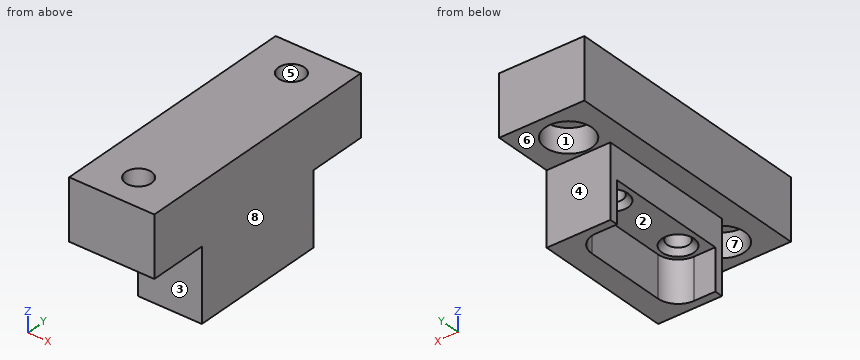
```python
from build123d import *

# Parameters (mm, degrees)
SKETCH2_W           = 16.5
SKETCH2_H           = 50
SKETCH2_R           = 2.5
BOSS_EXTRUDE1_DEPTH = 11.655
CUT_EXTRUDE3_START  = -7
SKETCH4_R           = 4.5
CUT_EXTRUDE3_DEPTH  = 10
SKETCH6_W           = 12.35
SKETCH6_H           = 27
BOSS_EXTRUDE2_DEPTH = 6
SKETCH7_R           = 2.1
CUT_EXTRUDE4_DEPTH  = 6
CHAMFER1_SIZE       = 1
BOSS_EXTRUDE3_DEPTH = 8


with BuildPart() as part:
    # Sketch2 → Boss-Extrude1 (new body)
    with BuildSketch(Plane.XY):
        with Locations((-2.723788813, 9.906715388)):
            Rectangle(SKETCH2_W, SKETCH2_H)
        with Locations((-2.723788813, -8.593284612)):
            Circle(SKETCH2_R, mode=Mode.SUBTRACT)
        with Locations((-2.723788813, 28.406715388)):
            Circle(SKETCH2_R, mode=Mode.SUBTRACT)
    extrude(amount=BOSS_EXTRUDE1_DEPTH)

    # Sketch4 → Cut-Extrude3 (cut)
    with BuildSketch(Plane.XY.offset(11.655).offset(CUT_EXTRUDE3_START)):
        with Locations((-2.723788813, 28.406715388)):
            Circle(SKETCH4_R)
        with Locations((-2.723788813, -8.593284612)):
            Circle(SKETCH4_R)
    extrude(amount=-CUT_EXTRUDE3_DEPTH, mode=Mode.SUBTRACT)

    # Sketch6 → Boss-Extrude2 (add)
    with BuildSketch(Plane(origin=(0, 0, 0), x_dir=(-1, 0, 0), z_dir=(0, 0, -1))):
        with Locations((0.648788813, 9.906715388)):
            Rectangle(SKETCH6_W, SKETCH6_H)
    extrude(amount=BOSS_EXTRUDE2_DEPTH)

    # Sketch7 → Cut-Extrude4 (cut)
    with BuildSketch(Plane(origin=(0, 0, -6), x_dir=(-1, 0, 0), z_dir=(0, 0, -1))):
        with Locations((2.723788813, 17.906715388)):
            Circle(SKETCH7_R)
        with Locations((2.723788813, 1.906715388)):
            Circle(SKETCH7_R)
    extrude(amount=-CUT_EXTRUDE4_DEPTH, mode=Mode.SUBTRACT)

    # Chamfer1
    chamfer1_edges = [part.edges().sort_by_distance(p)[0] for p in [
        (-0.623788813, 17.906715388, -6),
        (-0.623788813, 1.906715388, -6),
    ]]
    chamfer(chamfer1_edges, length=CHAMFER1_SIZE)

    # Sketch8 → Boss-Extrude3 (add)
    with BuildSketch(Plane(origin=(0, 0, -6), x_dir=(-1, 0, 0), z_dir=(0, 0, -1))):
        with BuildLine():
            Line((6.823788813, 21.806715388), (6.823788813, 23.406715388))
            Line((6.823788813, 23.406715388), (-5.526211187, 23.406715388))
            Line((-5.526211187, 23.406715388), (-5.526211187, -3.593284612))
            Line((-5.526211187, -3.593284612), (6.823788813, -3.593284612))
            Line((6.823788813, -3.593284612), (6.823788813, -1.993284612))
            Line((6.823788813, -1.993284612), (2.723788813, -1.993284612))
            ThreePointArc((2.723788813, -1.993284612), (-0.033927633, -0.851001059), (-1.176211187, 1.906715388))
            Line((-1.176211187, 1.906715388), (-1.176211187, 17.906715388))
            ThreePointArc((-1.176211187, 17.906715388), (-0.033927633, 20.664431835), (2.723788813, 21.806715388))
            Line((2.723788813, 21.806715388), (6.823788813, 21.806715388))
        make_face()
    extrude(amount=BOSS_EXTRUDE3_DEPTH)


solid = part.part
```
Work out the finished part from the listing and answer in its coordinate system (mm). Face numbers are marked on the shaded views. A direction names the side the tool comes from. Coordinates: 2 decimals unless noted, no trailing zeros. Loops run counter-clockwise (first coordinate to the right, second up) from the corner with the lowest first, then second, coordinate; pieces in that order, holes last.
1) Section C-C (y = 11) is taken. Give the vertices of the cut face in (x, z) (3 decimals).
Results:
outline: (-10.974, 0) - (-6.824, 0) - (-6.824, -6) - (1.176, -6) - (1.176, -14) - (5.526, -14) - (5.526, 11.655) - (-10.974, 11.655) - close
2) Consider probe 1 along Y at (x, z) = (-2.75, -1); probe 2 along Y at (x, z) = (-5, 3); probe 3 along Z at (x, y) = (-1.25, -5) (3 decimals). Determine where each line is inside the solid, lowest interval first.
Results:
probe 1: y = -3.59 to -0.19, 4.01 to 15.81, 20.01 to 23.41
probe 2: y = -15.09 to -12.48, -4.71 to 24.52, 32.29 to 34.91
probe 3: z = 4.655 to 11.655
3) Section A-A (z = -9.75) is taken. Give the vertices of the cut face in (x, y).
Results:
outline: (-6.82, -3.59) - (5.53, -3.59) - (5.53, 23.41) - (-6.82, 23.41) - (-6.82, 21.81) - (-2.72, 21.81) arc R3.9 cw to (1.18, 17.91) - (1.18, 1.91) arc R3.9 cw to (-2.72, -1.99) - (-6.82, -1.99) - close
4) For a pull along X with two mould halves and no side action, classify the marked faces 5, 6, 7 and 8 as +X half, -X half, draft (parallel to the pull), parting line (faces both ways), or undercut.
Results:
face 5: undercut
face 6: draft
face 7: undercut
face 8: +X half
5) Section D-D (z = -1) is taken. Give the vertices of the cut face in (x, y).
Results:
outline: (-6.82, -3.59) - (5.53, -3.59) - (5.53, 23.41) - (-6.82, 23.41) - close; hole circle Ø4.2 at (-2.72, 1.91); hole circle Ø4.2 at (-2.72, 17.91)
6) Flat-ended cylindrical pins translate along their axes: pin 1 (1.3 mm diameter, centred on x = -3, y = 17, fed in from -Z); pin 2 (2.5 mm diameter, centred on x = -2, y = -10.5, fed in from -Z) (3 decimals); pin 3 (6.5 mm diameter, centred on x = -2.72, y = 1.91, fed in from -Z); pin 4 (3 mm diameter, centred on x = -2.72, y = -8.59, fed in from +Z). Find the tip coordinate at first contact, or state that the pin passes through.
Results:
pin 1: stops at z = 0
pin 2: stops at z = 4.655
pin 3: stops at z = -6
pin 4: passes through
7) For the marked faces 1, 2, 3 and 4, determine the directions among +Z, -Z, +X, -X, +Y, -Y from which every point of the face is accessible in a straight line to the end or side of a thin tool.
Results:
face 1: -Z
face 2: -Z, -X
face 3: -Z, +X, -X, -Y
face 4: -Z, +X, -X, +Y
8) Section B-B (x = 2.75) is taken. Give the vertices of the cut face in (y, z) (3 decimals).
Results:
outline: (-15.093, 0) - (-3.593, 0) - (-3.593, -14) - (23.407, -14) - (23.407, 0) - (34.907, 0) - (34.907, 11.655) - (-15.093, 11.655) - close
